from build123d import *

# Parameters (mm, degrees)
SKETCH3_W               = 40
SKETCH3_H               = 50
BOSS_EXTRUDE1_DEPTH     = 5
SKETCH6_R               = 2.5
CUT_EXTRUDE6_DEPTH      = 41.620192023
SKETCH7_W               = 40
SKETCH7_H               = 5
BOSS_EXTRUDE2_DEPTH     = 15
SKETCH8_W               = 40
SKETCH8_H               = 28
BOSS_EXTRUDE3_DEPTH     = 3.9
CUT_EXTRUDE3_DEPTH      = 44.011626335
CUT_EXTRUDE3_DEPTH_BACK = 44.011626335
SKETCH1_R               = 6.5
SKETCH1_R_2             = 1.5
CUT_EXTRUDE7_REACH      = 57.227
SKETCH9_W               = 28
SKETCH9_H               = 3.9


with BuildPart() as part:
    # Sketch3 → Boss-Extrude1 (new body)
    with BuildSketch(Plane(origin=(0, 0, 0), x_dir=(1, 0, 0), z_dir=(0, 1, 0))):
        with Locations((0, -10)):
            Rectangle(SKETCH3_W, SKETCH3_H)
    extrude(amount=BOSS_EXTRUDE1_DEPTH)

    # Sketch6 → Cut-Extrude6 (cut, through all)
    with BuildSketch(Plane(origin=(0, 5, 0), x_dir=(1, 0, 0), z_dir=(0, 1, 0))):
        with Locations(Location((-12, -30, 0), (0, 0, 270))):
            Circle(SKETCH6_R)
        with Locations(Location((12, -30, 0), (0, 0, 270))):
            Circle(SKETCH6_R)
    extrude(amount=-CUT_EXTRUDE6_DEPTH, mode=Mode.SUBTRACT)

    # Sketch7 → Boss-Extrude2 (add)
    with BuildSketch(Plane.XZ):
        with Locations((0, 15.5)):
            Rectangle(SKETCH7_W, SKETCH7_H)
    extrude(amount=BOSS_EXTRUDE2_DEPTH)

    # Sketch8 → Boss-Extrude3 (add)
    with BuildSketch(Plane.XZ):
        with Locations((0, -1)):
            Rectangle(SKETCH8_W, SKETCH8_H)
    extrude(amount=BOSS_EXTRUDE3_DEPTH)

    # Sketch1 → Cut-Extrude3 (cut, two sides: drawn at the far end of the back side and taken through both)
    with BuildSketch(Plane(origin=(0, 0, 0), x_dir=(1, 0, 0), z_dir=(0, 1, 0)).offset(-CUT_EXTRUDE3_DEPTH_BACK)):
        with Locations(Location((0, 0, 0), (0, 0, 90))):
            Circle(SKETCH1_R)
        with Locations(Location((0, 8.6, 0), (0, 0, 90))):
            Circle(SKETCH1_R_2)
        with Locations(Location((0, -8.6, 0), (0, 0, 90))):
            Circle(SKETCH1_R_2)
    extrude(amount=CUT_EXTRUDE3_DEPTH + CUT_EXTRUDE3_DEPTH_BACK, mode=Mode.SUBTRACT)

    # Cut-Extrude7: up to this face of the body (flat: up to its plane)
    cut_extrude7_end = Plane(part.part.faces().sort_by_distance((20, -0.346476278, 8.183555965))[0])
    # Sketch9 → Cut-Extrude7 (cut, up to the picked face)
    with BuildSketch(Plane.ZY.offset(20), mode=Mode.PRIVATE) as cut_extrude7_sk1:
        with Locations((-1, 3.05)):
            Rectangle(SKETCH9_W, SKETCH9_H)
    cut_extrude7_tool1 = split(extrude(cut_extrude7_sk1.sketch, amount=-CUT_EXTRUDE7_REACH, mode=Mode.PRIVATE), bisect_by=cut_extrude7_end, keep=Keep.BOTH, mode=Mode.PRIVATE)
    add(cut_extrude7_tool1.solids().sort_by(Axis((-20, 3.05, -1), (1, 0, 0)))[0], mode=Mode.SUBTRACT)


solid = part.part
Model file for the job. Use its own axes, mm. A direction names the side the tool comes from. Give positions to 0.01 mm unless a question says otherwise; leave off trailing zeros. Loops run counter-clockwise (first coordinate to the right, second up) from the corner with the lowest first, then second, coordinate; pieces in that order, holes last.
1) Tool access for faces 1 (the cylindrical face through (0.575, -1.435, -9.986)), 2 (the flat face through (0, -7, 18)), 3 (the flat face through (0, -9, 13)), 4 (the flat face through (4, 1.1, -7)): list every direction of +Z, -Z, +X, -X, +Y, -Y with a clear straight run to the whole face (end or side of a thin tool).
2) Saw through at B-B (x = -12). Write the cut outline in (y, z).
3) Saw through at D-D (y = -0.75). Write the cut outline in (x, z).
4) Wall check: line 1 (X direction, y = 1.4, z = 30); line 2 (X direction, y = -2.1, z = -8.6); line 3 (Y direction, x = 17.5, z = 2.5). Give the ranges that are in metal, low to high.
5) Pull direction Z, two halves, no side cores. Call faces 5 (the cylindrical face through (-13.5, 2.5, 28)), 6 (the flat face through (0, 5, 24)), 7 (the cylindrical face through (9.56, 2.54, 29.46)), 8 (the flat face through (0, -1, -15)): +Z half, -Z half, draft (parallel to the pull), parting line (faces both ways), or undercut.
6) Saw through at A-A (z = 8.6). Write the cut outline in (x, y).
7) Saw through at C-C (z = 30). Write the cut outline in (x, y), plus the area to 3 significant figures.
8) Flat gauge pins, fed straight in: pin 1 Ø14 at (x, z) = (0, -7.5) entering from +Y; pin 2 Ø2 at (x, y) = (-1, 3.5) entering from -Z; pin 3 Ø5 at (x, z) = (8, 28) entering from -Y. Where does each tip first touch, or does it go through?
Answer block:
1. face 1: +Y, -Y
1. face 2: +Z, +X, -X, -Y
1. face 3: -Z, +X, -X, -Y
1. face 4: -Z, +X, -X, +Y
2. outline: (-15, 13) - (-3.9, 13) - (-3.9, -15) - (1.1, -15) - (1.1, 13) - (5, 13) - (5, 27.5) - (0, 27.5) - (0, 18) - (-15, 18) - close; (0, 32.5) - (5, 32.5) - (5, 35) - (0, 35) - close
3. outline: (-20, -15) - (20, -15) - (20, 18) - (-20, 18) - close; hole circle Ø13 at (0, 0); hole circle Ø3 at (0, -8.6); hole circle Ø3 at (0, 8.6)
4. line 1: x = -20 to -14.5, -9.5 to 9.5, 14.5 to 20
4. line 2: x = -20 to -1.5, 1.5 to 20
4. line 3: y = -3.9 to 1.1
5. face 5: undercut
5. face 6: draft
5. face 7: undercut
5. face 8: -Z half
6. outline: (-20, -3.9) - (-1.5, -3.9) - (-1.5, 1.1) - (-20, 1.1) - close; (1.5, -3.9) - (20, -3.9) - (20, 1.1) - (1.5, 1.1) - close
7. outline: (-20, 0) - (-14.5, 0) - (-14.5, 5) - (-20, 5) - close; (-9.5, 0) - (9.5, 0) - (9.5, 5) - (-9.5, 5) - close; (14.5, 0) - (20, 0) - (20, 5) - (14.5, 5) - close
7. area: 150 mm2
8. pin 1: stops at y = 1.1
8. pin 2: stops at z = 13
8. pin 3: stops at y = 0
